from build123d import *

# Parameters (mm, degrees)
SKETCH1_W           = 40
SKETCH1_H           = 25
SKETCH1_R           = 1
BOSS_EXTRUDE1_DEPTH = 5
SKETCH2_W           = 15
SKETCH2_H           = 5
BOSS_EXTRUDE2_DEPTH = 40
FILLET2_R           = 10
SKETCH8_R           = 1.5
CUT_EXTRUDE1_DEPTH  = 40


with BuildPart() as part:
    # Sketch1 → Boss-Extrude1 (new body)
    with BuildSketch(Plane.XY):
        with Locations((20, 12.5)):
            Rectangle(SKETCH1_W, SKETCH1_H)
        with Locations((11, 23)):
            Circle(SKETCH1_R, mode=Mode.SUBTRACT)
        with Locations((29, 23)):
            Circle(SKETCH1_R, mode=Mode.SUBTRACT)
    extrude(amount=BOSS_EXTRUDE1_DEPTH)

    # Sketch2 → Boss-Extrude2 (add)
    with BuildSketch(Plane.ZY):
        with Locations((-7.5, 2.5)):
            Rectangle(SKETCH2_W, SKETCH2_H)
    extrude(amount=-BOSS_EXTRUDE2_DEPTH)

    # Fillet2
    fillet2_edges = [part.edges().sort_by_distance(p)[0] for p in [
        (20, 5, 0),
    ]]
    fillet(fillet2_edges, radius=FILLET2_R)

    # Sketch8 → Cut-Extrude1 (cut)
    with BuildSketch(Plane(origin=(0, 0, 0), x_dir=(-1, 0, 0), z_dir=(0, -1, 0))):
        with Locations((-6.5, 12.5)):
            Circle(SKETCH8_R)
        with Locations((-33.5, 12.5)):
            Circle(SKETCH8_R)
    extrude(amount=-CUT_EXTRUDE1_DEPTH, mode=Mode.SUBTRACT)


solid = part.part
Build history of the part. All positions in model axes, mm. A direction names the side the tool comes from. Coordinates: 2 decimals unless noted, no trailing zeros. Write each loop counter-clockwise with the first axis right and the second up, starting at its lowest first coordinate (ties: lowest second). Pieces come first, ordered by that corner, then holes.
(1) Drill centre lines: line 1 (X direction, y = 1.4, z = -12.5); line 2 (Y direction, x = 29, z = 1.15); line 3 (Z direction, x = 33.5, y = 2.05). Where is each one in solid material? Low to high.
(2) Mould opens along Z. For faces 3 (the cylindrical face through (7.7, 2.5, -11.6)), 4 (the flat face through (0, 7, -1)), 5 (the flat face through (20, 20, 0)) say: pulls with the +Z half, pulls with the -Z half, needs draft (parallel to the pull), parting line crosses it, or undercut.
(3) Cut at C-C on x = 33.5. List the corners of the cut face in (y, z), and give its area (3 significant figures).
(4) Cut at D-D on x = 13. List the corners of the cut face in (y, z), and give its area (3 significant figures).
(5) Pin check, flat tips, straight feed: pin 1 Ø3 at (x, y) = (19.5, 18) entering from -Z; pin 2 Ø10 at (x, z) = (29.5, -4.5) entering from +Y; pin 3 Ø3.5 at (x, z) = (33.5, -12.5) entering from +Y; pin 4 Ø8 at (x, z) = (6.5, -5) entering from +Y. Stop position of each tip, or through.
(6) Cut at B-B on z = -12.5. List the corners of the cut face in (x, y), and give its area (3 significant figures).
(7) 3-axis set-ups, long thin cutter, end or side, ignore diameter. For faces 1 (the flat face through (20, 5, -13)), 2 (the cylindrical face through (34.7, 2.5, -11.6)): which of +Z, -Z, +X, -X, +Y, -Y reach the whole face in a straight line?
(8) Cut at A-A on y = 23. List the corners of the cut face in (x, z), and give its area (3 significant figures).
Working result:
1. line 1: x = 0 to 5, 8 to 32, 35 to 40
1. line 2: y = 0 to 22, 24 to 25
1. line 3: z = -15 to -14, -11 to 5
2. face 3: undercut
2. face 4: needs draft
2. face 5: pulls with the -Z half
3. outline: (0, -15) - (5, -15) - (5, -14) - (0, -14) - close; (0, -11) - (5, -11) - (5, -10) arc R10 cw to (15, 0) - (25, 0) - (25, 5) - (0, 5) - close
3. area: 206 mm2
4. outline: (0, -15) - (5, -15) - (5, -10) arc R10 cw to (15, 0) - (25, 0) - (25, 5) - (0, 5) - close
4. area: 221 mm2
5. pin 1: stops at z = 0
5. pin 2: stops at y = 25
5. pin 3: stops at y = 5
5. pin 4: stops at y = 10.64
6. outline: (0, 0) - (5, 0) - (5, 5) - (0, 5) - close; (8, 0) - (32, 0) - (32, 5) - (8, 5) - close; (35, 0) - (40, 0) - (40, 5) - (35, 5) - close
6. area: 170 mm2
7. face 1: -Z, +X, -X, +Y
7. face 2: +Y, -Y
8. outline: (0, 0) - (10, 0) - (10, 5) - (0, 5) - close; (12, 0) - (28, 0) - (28, 5) - (12, 5) - close; (30, 0) - (40, 0) - (40, 5) - (30, 5) - close
8. area: 180 mm2
